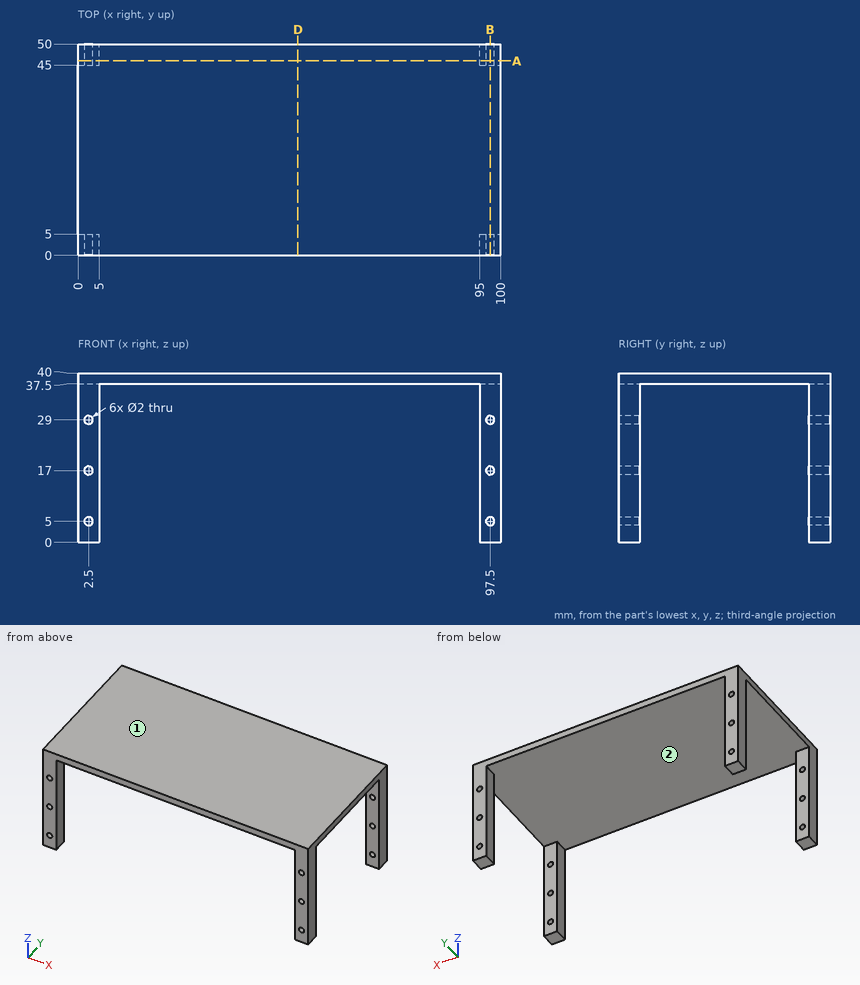
Input: dimensioned drawing with shaded views. Units: mm. Origin: part minimum x, y, z. Round coordinates to 2 decimals unless told otherwise and drop trailing zeros. Order: outer loops, then holes, each group sorted by start corner. A loop starts at its lowest first (then second) coordinate and runs counter-clockwise, first axis right, second up.
1. Cut plane D-D, the plane x = 52. Output: boundary loops of the cut face in (y, z), then the cut area to 3 significant figures.
The answers:
outline: (0, 37.5) - (50, 37.5) - (50, 40) - (0, 40) - close
area: 125 mm2
2. Cut plane B-B, the plane x = 97.5. State how many separate pieces and enclosed holes the cut face has, then the cut area to 3 significant figures.
The answers:
separate pieces: 7
enclosed holes: 0
area: 440 mm2
3. Pin query (flat end, axial travel): P1, Ø5, axis at x = 24, y = 35, coming from the -Z side; P2, Ø4, axis at y = 47.5, z = 25.5, coming from the -X side. Return the tip coordinate at first contact, or that it passes through.
The answers:
P1: stops at z = 37.5
P2: stops at x = 0
4. Material intervals for line 1 (Z direction, x = 97.5, y = 2.95); line 2 (X direction, y = 46, z = 12); line 3 (Z direction, x = 38.5, y = 26), sorted ascending.
The answers:
line 1: z = 0 to 4, 6 to 16, 18 to 28, 30 to 40
line 2: x = 0 to 5, 95 to 100
line 3: z = 37.5 to 40
5. Cut plane A-A, the plane y = 46. Output: boundary loops of the cut face in (x, z).
The answers:
outline: (0, 0) - (5, 0) - (5, 37.5) - (95, 37.5) - (95, 0) - (100, 0) - (100, 40) - (0, 40) - close; hole circle Ø2 at (2.5, 5); hole circle Ø2 at (2.5, 17); hole circle Ø2 at (2.5, 29); hole circle Ø2 at (97.5, 5); hole circle Ø2 at (97.5, 17); hole circle Ø2 at (97.5, 29)
6. Mould query, pull axis X, two halves, no side actions, for the marked faces 1 and 2. Classes: released by +X, released by -X, zero draft, split by the parting line, or undercut.
The answers:
face 1: zero draft
face 2: undercut
